For this review, take the finished solid that the model builds, in its own axes (mm). A direction names the side the tool comes from. Coordinates: 2 decimals unless noted, no trailing zeros. Write each loop counter-clockwise with the first axis right and the second up, starting at its lowest first coordinate (ties: lowest second). Pieces come first, ordered by that corner, then holes. Notation, with made-up numbers: M -35.75,54.25 L 4.25,54.25 A33 ccw 4.25,92.25 Z; hole C -20.75,65 d2. An arc over 180 degrees is marked long. Return JSON: item names as keys, results as strings.
```python
from build123d import *

# Parameters (mm, degrees)
BOSS_EXTRUDE1_DEPTH     = 5
BOSS_EXTRUDE2_DEPTH     = 5
BOSS_EXTRUDE3_DEPTH     = 5
SKETCH6_R               = 2.5
CUT_EXTRUDE1_DEPTH      = 107.549284371
SKETCH9_R               = 4.1275
SKETCH9_R_2             = 2.6035
BOSS_EXTRUDE5_DEPTH     = 35.56
FILLET1_R               = 0.508
BOSS_EXTRUDE6_DEPTH     = 19.05
SKETCH15_R              = 2.38125
BOSS_EXTRUDE7_DEPTH     = 15.875
CHAMFER2_SIZE           = 7.62
FILLET2_R               = 1.27
SKETCH16_W              = 7.844007501
SKETCH16_H              = 4.112882263
BOSS_EXTRUDE8_DEPTH     = 3.175
CHAMFER3_SIZE           = 1.27
SKETCH17_R              = 1.984375
SKETCH17_R_2            = 1.9288125
BOSS_EXTRUDE9_DEPTH     = 16.51
CUT_EXTRUDE2_REACH      = 111.603
SKETCH18_R              = 2.38125
CUT_EXTRUDE3_REACH      = 111.603
SKETCH19_R              = 2.38125
CUT_EXTRUDE4_DEPTH      = 4.13271
CUT_EXTRUDE4_DEPTH_BACK = 1.27
CUT_EXTRUDE5_DEPTH      = 1.27


with BuildPart() as part:
    # Sketch1 → Boss-Extrude1 (new body)
    with BuildSketch(Plane(origin=(0, 0, 0), x_dir=(1, 0, 0), z_dir=(0, 1, 0))):
        Polygon((0, 0), (0, 60.5), (60.5, 60.5), (60.5, 47.75), (12.75, 0), align=None)
    extrude(amount=BOSS_EXTRUDE1_DEPTH)

    # Sketch4 → Boss-Extrude2 (add)
    with BuildSketch(Plane.ZY):
        Polygon((-60.5, 5), (-60.5, 68.5), (-19.4, 68.5), (0, 10.308629506), (0, 5), align=None)
    extrude(amount=-BOSS_EXTRUDE2_DEPTH)

    # Sketch5 → Boss-Extrude3 (add)
    with BuildSketch(Plane(origin=(0, 0, -60.5), x_dir=(-1, 0, 0), z_dir=(0, 0, -1))):
        Polygon((-5, 5), (-5, 68.5), (-41, 68.5), (-60.5, 10.004653177), (-60.5, 5), align=None)
    extrude(amount=-BOSS_EXTRUDE3_DEPTH)

    # Sketch6 → Cut-Extrude1 (cut, through all)
    with BuildSketch(Plane(origin=(0, 5, 0), x_dir=(1, 0, 0), z_dir=(0, 1, 0))):
        with Locations(Location((16.5, 15, 0), (0, 0, 270))):
            Circle(SKETCH6_R)
        with Locations(Location((45.5, 44.625, 0), (0, 0, 270))):
            Circle(SKETCH6_R)
    extrude(amount=-CUT_EXTRUDE1_DEPTH, mode=Mode.SUBTRACT)

    # Sketch9 → Boss-Extrude5 (add)
    with BuildSketch(Plane.XY.offset(-55.5)):
        with Locations(Location((49.45, 19.0462, 0), (0, 0, 180))):
            Circle(SKETCH9_R)
        with Locations(Location((49.45, 19.0462, 0), (0, 0, 180))):
            Circle(SKETCH9_R_2, mode=Mode.SUBTRACT)
    extrude(amount=BOSS_EXTRUDE5_DEPTH)

    # Fillet1
    fillet1_edges = [part.edges().sort_by_distance(p)[0] for p in [
        (52.0535, 19.0462, -19.94),
    ]]
    fillet(fillet1_edges, radius=FILLET1_R)

    # Sketch14 → Boss-Extrude6 (add)
    with BuildSketch(Plane(origin=(0, 5, 0), x_dir=(1, 0, 0), z_dir=(0, 1, 0))):
        with BuildLine():
            Line((6.722962691, 28.802730135), (9.132707699, 31.364136576))
            ThreePointArc((9.132707699, 31.364136576), (10.457950503, 50.042049497), (29.135863424, 51.367292301))
            Line((29.135863424, 51.367292301), (31.697269865, 53.777037309))
            ThreePointArc((31.697269865, 53.777037309), (36.686417723, 53.662894944), (36.648367319, 48.672586637))
            Line((36.648367319, 48.672586637), (33.860208422, 45.884427741))
            ThreePointArc((33.860208422, 45.884427741), (34.790141211, 43.96666613), (35.539002262, 41.971223395))
            Line((35.539002262, 41.971223395), (35.799607225, 42.077391474))
            Line((35.799607225, 42.077391474), (35.633459083, 42.367636838))
            ThreePointArc((35.633459083, 42.367636838), (35.320181387, 43.965693178), (36.041784088, 45.425561844))
            Line((36.041784088, 45.425561844), (38.110219678, 47.493997435))
            ThreePointArc((38.110219678, 47.493997435), (38.110219678, 54.843851927), (30.760365187, 54.843851927))
            Line((30.760365187, 54.843851927), (28.830026438, 52.913513178))
            ThreePointArc((28.830026438, 52.913513178), (8.980759009, 50.993661336), (7.060907167, 31.144393908))
            Line((7.060907167, 31.144393908), (5.656148073, 29.739634813))
            ThreePointArc((5.656148073, 29.739634813), (5.656148073, 22.389780322), (13.006002565, 22.389780322))
            Line((13.006002565, 22.389780322), (15.074438156, 24.458215912))
            ThreePointArc((15.074438156, 24.458215912), (15.744974902, 24.939184047), (16.534306822, 25.179818613))
            Line((16.534306822, 25.179818613), (16.568898656, 25.694636548))
            ThreePointArc((16.568898656, 25.694636548), (15.581109404, 26.144220149), (14.615572259, 26.639791578))
            Line((14.615572259, 26.639791578), (11.827413363, 23.851632681))
            ThreePointArc((11.827413363, 23.851632681), (6.837105056, 23.813582277), (6.722962691, 28.802730135))
        make_face()
    extrude(amount=BOSS_EXTRUDE6_DEPTH)

    # Sketch15 → Boss-Extrude7 (add)
    with BuildSketch(Plane(origin=(0, 68.5, 0), x_dir=(1, 0, 0), z_dir=(0, 1, 0))):
        Polygon((5, 55.5), (5, 30.3375), (30.1625, 55.5), align=None)
        with Locations(Location((9.525, 50.975, 0), (0, 0, 270))):
            Circle(SKETCH15_R, mode=Mode.SUBTRACT)
    extrude(amount=-BOSS_EXTRUDE7_DEPTH)

    # Chamfer2
    chamfer2_edges = [part.edges().sort_by_distance(p)[0] for p in [
        (17.58125, 52.625, -42.91875),
    ]]
    chamfer(chamfer2_edges, length=CHAMFER2_SIZE)

    # Fillet2
    fillet2_edges = [part.edges().sort_by_distance(p)[0] for p in [
        (15.744974902, 5, -24.939184047),
        (14.04022036, 5, -23.423998117),
        (8.812852099, 5, -20.893477035),
        (35.320181387, 5, -43.965693178),
        (35.716533154, 5, -42.222514156),
        (37.076001883, 5, -46.45977964),
        (39.606522965, 5, -51.687147901),
    ]]
    fillet(fillet2_edges, radius=FILLET2_R)

    # Sketch16 → Boss-Extrude8 (add)
    with BuildSketch(Plane.XY.offset(-55.5)):
        with Locations((42.208447341, 21.154254949)):
            Rectangle(SKETCH16_W, SKETCH16_H)
    extrude(amount=BOSS_EXTRUDE8_DEPTH)

    # Chamfer3
    chamfer3_edges = [part.edges().sort_by_distance(p)[0] for p in [
        (38.28644359, 23.21069608, -55.07937031),
    ]]
    chamfer(chamfer3_edges, length=CHAMFER3_SIZE)

    # Sketch17 → Boss-Extrude9 (add)
    # profile 1 of 2: a face of its own
    with BuildSketch(Plane(origin=(0, 5, 0), x_dir=(1, 0, 0), z_dir=(0, 1, 0))):
        with BuildLine():
            Line((14.046968971, 26.071188289), (8.715956726, 30.921156666))
            Line((8.715956726, 30.921156666), (6.722962691, 28.802730135))
            ThreePointArc((6.722962691, 28.802730135), (6.837105056, 23.813582277), (11.827413363, 23.851632681))
            Line((11.827413363, 23.851632681), (14.046968971, 26.071188289))
        make_face()
        with Locations(Location((10.020377911, 27.007841876, 0), (0, 0, 90))):
            Circle(SKETCH17_R, mode=Mode.SUBTRACT)
    # profile 2 of 2: a face of its own
    with BuildSketch(Plane(origin=(0, 5, 0), x_dir=(1, 0, 0), z_dir=(0, 1, 0))):
        with BuildLine():
            Line((31.697269865, 53.777037309), (29.66316707, 51.863374183))
            Line((29.66316707, 51.863374183), (34.595934869, 46.620154187))
            Line((34.595934869, 46.620154187), (36.648367319, 48.672586637))
            ThreePointArc((36.648367319, 48.672586637), (36.686417723, 53.662894944), (31.697269865, 53.777037309))
        make_face()
        with Locations(Location((33.690847255, 50.732351927, 0), (0, 0, 90))):
            Circle(SKETCH17_R_2, mode=Mode.SUBTRACT)
    extrude(amount=BOSS_EXTRUDE9_DEPTH)

    # Sketch18 → Cut-Extrude2 (cut, up to next)
    with BuildSketch(Plane.ZY, mode=Mode.PRIVATE) as cut_extrude2_sk1:
        with Locations((-32.56, 49.53)):
            Circle(SKETCH18_R)
    cut_extrude2_tool1 = extrude(cut_extrude2_sk1.sketch, amount=-CUT_EXTRUDE2_REACH, mode=Mode.PRIVATE) & part.part
    add(cut_extrude2_tool1.solids().sort_by_distance((0, 49.53, -32.56))[0], mode=Mode.SUBTRACT)

    # Sketch19 → Cut-Extrude3 (cut, up to next)
    with BuildSketch(Plane(origin=(0, 0, -60.5), x_dir=(-1, 0, 0), z_dir=(0, 0, -1)), mode=Mode.PRIVATE) as cut_extrude3_sk1:
        with Locations((-27.78125, 26.19375)):
            Circle(SKETCH19_R)
    cut_extrude3_tool1 = extrude(cut_extrude3_sk1.sketch, amount=-CUT_EXTRUDE3_REACH, mode=Mode.PRIVATE) & part.part
    add(cut_extrude3_tool1.solids().sort_by_distance((27.78125, 26.19375, -60.5))[0], mode=Mode.SUBTRACT)

    # Sketch20 → Cut-Extrude4 (cut, two sides: drawn at the far end of the back side and taken through both)
    with BuildSketch(Plane.XY.offset(-55.5).offset(-CUT_EXTRUDE4_DEPTH_BACK)):
        Polygon((31.447424209, 26.19375), (29.614337105, 29.36875), (25.948162895, 29.36875), (24.115075791, 26.19375), (25.948162895, 23.01875), (29.614337105, 23.01875), align=None)
    extrude(amount=CUT_EXTRUDE4_DEPTH + CUT_EXTRUDE4_DEPTH_BACK, mode=Mode.SUBTRACT)

    # Sketch21 → Cut-Extrude5 (cut)
    with BuildSketch(Plane(origin=(5, 0, 0), x_dir=(0, 0, -1), z_dir=(1, 0, 0))):
        Polygon((34.393087105, 52.705), (30.726912895, 52.705), (28.893825791, 49.53), (30.726912895, 46.355), (34.393087105, 46.355), (36.226174209, 49.53), align=None)
    extrude(amount=-CUT_EXTRUDE5_DEPTH, mode=Mode.SUBTRACT)


solid = part.part
```
1. We need section C-C (x = 49.45). State the section outline as (y, z) points, plus the area to 3 significant figures.
Checks:
{"outline": "M 0,-60.5 L 43.15,-60.5 L 43.15,-55.5 L 23.17,-55.5 L 23.17,-19.94 L 22.16,-19.94 A0.51 ccw 21.65,-20.45 L 21.65,-55.5 L 16.44,-55.5 L 16.44,-20.45 A0.51 ccw 15.93,-19.94 L 14.92,-19.94 L 14.92,-55.5 L 5,-55.5 L 5,-36.7 L 0,-36.7 Z", "area": "418 mm2"}
2. Clearance check with flat-ended pins moving along their axes: pin 1 Ø2 at (x, z) = (11, -27.5) entering from +Y; pin 2 Ø7.5 at (y, z) = (49.53, -32.56) entering from +X; pin 3 Ø10.5 at (x, z) = (36.5, -50) entering from +Y; pin 4 Ø8 at (x, z) = (44.5, -14.5) entering from -Y. State where each tip first meets the part, or that it passes through.
Checks:
{"pin 1": "y = 21.51", "pin 2": "x = 5", "pin 3": "y = 24.05", "pin 4": "through"}
3. Wall thickness on L1, parallel to Y at x = 49.45, z = -40; L2, parallel to Y at x = 9, z = -46.5 (3 decimals); L3, parallel to Z at x = 39, y = 44: over which ranges is each line inside the solid? List them lowest first. Write a range as from..to.
Checks:
{"L1": "0..5, 14.92..16.44, 21.65..23.17", "L2": "0..5, 52.625..68.5", "L3": "-60.5..-55.5"}
4. For faces 3 (the face through (8, 21.51, -26)), 4 (the face through (4.4, 51.1, -29.8)), 5 (the face through (5, 30, -27)), list the 3-axis set-ups (+Z, -Z, +X, -X, +Y, -Y) from which the entire face can be reached by the end or side of a thin tool; tool diameter is ignored.
Checks:
{"face 3": "+Y", "face 4": "+X", "face 5": "none"}
5. We need section B-B (z = -15). State the section outline as (x, y) points.
Checks:
{"outline": "M 0,0 L 14,0 L 14,5 L 5,5 L 5,55.3 L 0,55.3 Z; M 19,0 L 27.75,0 L 27.75,5 L 19,5 Z"}
6. Draft analysis for pull direction X (two halves, no side actions). For faces 1 (the face through (43, 23.211, -54)), 2 (the face through (49, 19, -55.5)), state which applies: +X half, -X half, draft (parallel to the pull), parting line (faces both ways), or undercut.
Checks:
{"face 1": "draft", "face 2": "undercut"}
7. We need section A-A (z = -37.5). Give the number of separate pieces and of enclosed holes in the cut face, plus the area to 3 significant figures.
Checks:
{"separate pieces": "2", "enclosed holes": "1", "area": "706 mm2"}
